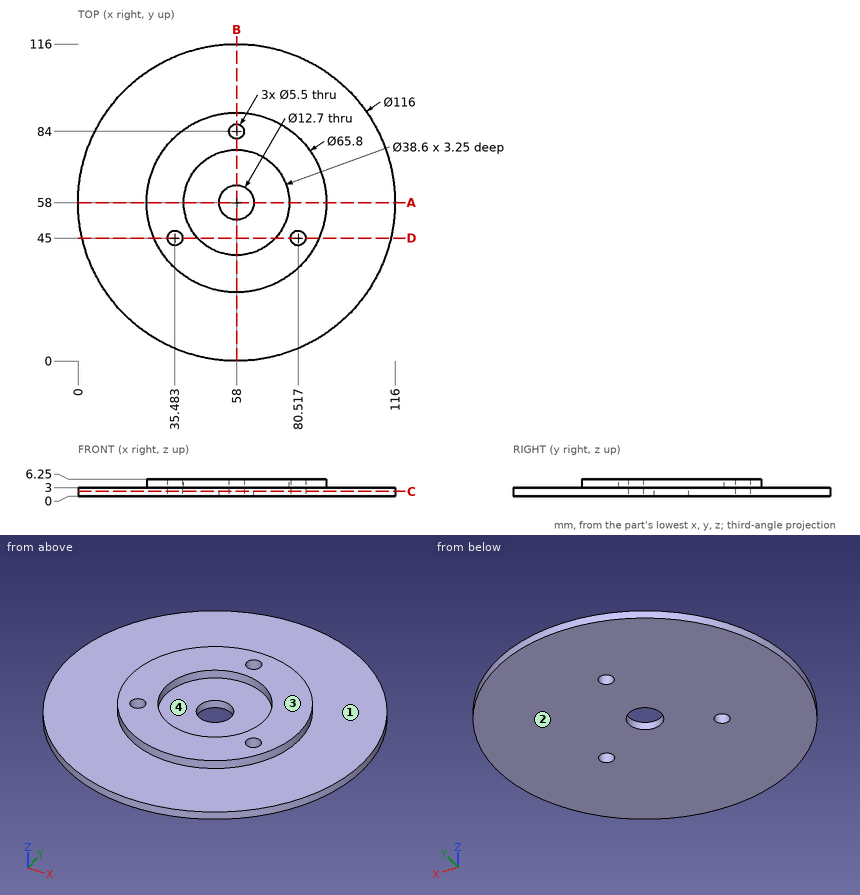
Answer from the drawing. Dimensions are ordinates in mm from the lowest x, y and z of the part. A direction names the side the tool comes from. Give positions to 0.01 mm unless a question says otherwise; leave off trailing zeros. Loops run counter-clockwise (first coordinate to the right, second up) from the corner with the lowest first, then second, coordinate; pieces in that order, holes last.
Item 1: The part is cut by section B-B (x = 58). Write down the section's boundary in (y, z).
Item 2: The mould has two halves that part along X. Classify the marked faces 3 and 4: released by +X, released by -X, zero draft, split by the parting line, or undercut.
Item 3: For the marked faces 1 and 2, determine the directions among +Z, -Z, +X, -X, +Y, -Y from which every point of the face is accessible in a straight line to the end or side of a thin tool.
Item 4: Find the intervals of material crossed by line 1 along Y through (x, z) = (58, 1.15); line 2 along Y through (x, z) = (58, 4.75); line 3 along X through (y, z) = (58, 4.15), in increasing order.
Item 5: Each of these flat-tipped pins is pushed along its axis until it touches: pin 1 Ø1 at (y, z) = (98, 1) entering from -X; pin 2 Ø3 at (x, y) = (17, 74) entering from +Z; pin 3 Ø1 at (y, z) = (37.5, 2.5) entering from -X. Where does it stop, or does it pass through?
Item 6: The part is cut by section C-C (z = 1.75). Write down the section's boundary in (x, y), and give its area (3 significant figures).
Item 7: The part is cut by section A-A (y = 58). Write down the section's boundary in (x, z), and give its area (3 significant figures).
Item 8: The part is cut by section D-D (y = 45). Give the number of separate pieces and of enclosed holes in the cut face, and give its area (3 significant figures).
Taken from the geometry:
1. outline: (0, 0) - (51.65, 0) - (51.65, 3) - (38.7, 3) - (38.7, 6.25) - (25.1, 6.25) - (25.1, 3) - (0, 3) - close; (64.35, 0) - (81.25, 0) - (81.25, 6.25) - (77.3, 6.25) - (77.3, 3) - (64.35, 3) - close; (86.75, 0) - (116, 0) - (116, 3) - (90.9, 3) - (90.9, 6.25) - (86.75, 6.25) - close
2. face 3: zero draft
2. face 4: undercut
3. face 1: +Z
3. face 2: -Z, +X, -X, +Y, -Y
4. line 1: y = 0 to 51.65, 64.35 to 81.25, 86.75 to 116
4. line 2: y = 25.1 to 38.7, 77.3 to 81.25, 86.75 to 90.9
4. line 3: x = 25.1 to 38.7, 77.3 to 90.9
5. pin 1: stops at x = 15.53
5. pin 2: stops at z = 3
5. pin 3: stops at x = 3.56
6. outline: circle Ø116 at (58, 58); hole circle Ø5.5 at (35.48, 45); hole circle Ø12.7 at (58, 58); hole circle Ø5.5 at (58, 84); hole circle Ø5.5 at (80.52, 45)
6. area: 10,400 mm2
7. outline: (0, 0) - (51.65, 0) - (51.65, 3) - (38.7, 3) - (38.7, 6.25) - (25.1, 6.25) - (25.1, 3) - (0, 3) - close; (64.35, 0) - (116, 0) - (116, 3) - (90.9, 3) - (90.9, 6.25) - (77.3, 6.25) - (77.3, 3) - (64.35, 3) - close
7. area: 398 mm2
8. separate pieces: 3
8. enclosed holes: 0
8. area: 374 mm2
